Autodesk Inventor part; units mm, degrees
ref_plane "YZ Plane" through (0, 0, 0) normal (1, 0, 0) x (0, 1, 0)
ref_plane "XZ Plane" through (0, 0, 0) normal (0, 1, 0) x (-1, 0, 0)
ref_plane "XY Plane" through (0, 0, 0) normal (0, 0, 1) x (1, 0, 0)
sketch "Esboço1" plane through (0, 0, 0) normal (0, 0, 1) x (1, 0, 0)
  line L0 (0, 0) -> (75, 0)
  line L1 (75, 0) -> (75, 3)
  line L2 (75, 3) -> (0, 3)
  line L3 (0, 3) -> (0, 0)
  dimension "d0" = 75
  dimension "d1" = 3
revolve "Revolução1" add sketch "Esboço1" angle 360 about axis through (0, 0, 0) along (1, 0, 0)
sketch "Esboço2" plane through (0, 0, 0) normal (0, 1, 0) x (-1, 0, 0)
  point P0 (0, 0)
chamfer "Chanfro1" distance 0.5 angle 45 2 edges at (0, -3, 0) (75, -3, 0)
sketch "Esboço3" plane through (0, 0, 0) normal (0, 1, 0) x (-1, 0, 0)
  line L0 (0, 2.5) -> (0, -2.5)
  line L1 (-75, 2.5) -> (-74.5, 3)
  line L2 (-74.5, 3) -> (-0.5, 3)
  line L3 (-0.5, 3) -> (0, 2.5)
  line L4 (0, 2.5) -> (0, -2.5)
  line L5 (0, -2.5) -> (-0.5, -3)
  line L6 (-0.5, -3) -> (-74.5, -3)
  line L7 (-74.5, -3) -> (-75, -2.5)
  line L8 (-75, -2.5) -> (-75, 2.5)
  arc A0 (-9.5, -2) -> (-14.5, -2) centre (-12, -2) ccw
  line L9 (-65.5, 2) -> (-65.5, 3)
  line L10 (-60.5, 3) -> (-60.5, 2)
  arc A1 (-60.7087, 3) -> (-65.2913, 3) centre (-63, 2) ccw
  arc A2 (-65.5, 2) -> (-60.5, 2) centre (-63, 2) ccw
  line L11 (-65.5, 3) -> (-65.2913, 3)
  line L12 (-60.7087, 3) -> (-60.5, 3)
  line L13 (-75, 2.5) -> (-74.5, 3)
  line L14 (-74.5, 3) -> (-0.5, 3)
  line L15 (-0.5, 3) -> (0, 2.5)
  line L16 (0, 2.5) -> (0, -2.5)
  line L17 (0, -2.5) -> (-0.5, -3)
  line L18 (-0.5, -3) -> (-74.5, -3)
  line L19 (-74.5, -3) -> (-75, -2.5)
  line L20 (-75, -2.5) -> (-75, 2.5)
  line L21 (-0.5, -3) -> (-0.5, 3)
  line L22 (-74.5, 3) -> (-74.5, -3)
  line L23 (-75, 2.5) -> (-74.5, 3)
  line L24 (-74.5, 3) -> (-0.5, 3)
  line L25 (-0.5, 3) -> (0, 2.5)
  line L26 (0, 2.5) -> (0, -2.5)
  line L27 (0, -2.5) -> (-0.5, -3)
  line L28 (-0.5, -3) -> (-74.5, -3)
  line L29 (-74.5, -3) -> (-75, -2.5)
  line L30 (-75, -2.5) -> (-75, 2.5)
  line L31 (-14.5, -2) -> (-14.5, -5)
  line L32 (-14.5, -5) -> (-9.5, -5)
  line L33 (-9.5, -5) -> (-9.5, -2)
  point P0 (0, 0)
  point P1 (-14.5, -3)
  point P2 (-9.5, -3)
  point P3 (-14.5, -3)
  point P4 (-9.5, -3)
  dimension "d10" = 12
  dimension "d12" = 12
  dimension "d17" = 2.5
  dimension "d19" = 5
  dimension "d20" = 3
  dimension "d21" = 1
extrude "Extrusão1" cut sketch "Esboço3" against normal mid plane 1 contours L10 A2 L9 L2 | L6 L31 A0 L33 | L2 A1
properties part number "Mainpulo"
Geometry check sheet. Reference: the model listing, model coordinates, mm. A direction names the side the tool comes from. Coordinates: 2 decimals unless noted, no trailing zeros. Loops run counter-clockwise (first coordinate to the right, second up) from the corner with the lowest first, then second, coordinate; pieces in that order, holes last. Notation, with made-up numbers: (23.5, -29) - (77.5, -29) arc R18 ccw to (77.5, -13) - close; hole circle Ø4 at (48, 52). An arc over 180 degrees is marked (long way). One line per item, written item: value. Start each with the question number.
(1) Cross-section at A-A on x = 63. Enter the section's corners in (y, z).
(2) Cross-section at B-B on x = 50. Enter the section's corners in (y, z), plus the area to 3 significant figures.
(3) Material ranges on line 1 (Z direction, x = 52, y = -0.45); line 2 (Y direction, x = 26.5, z = 0.5); line 3 (X direction, y = -0.2, z = 1), recorded low to high. Write a range as [from, to].
(4) Depth check by flat-ended pin: P1, Ø1.5, axis at x = 37.5, z = 2, coming from the +Y side; P2, Ø3, axis at x = 37.5, z = -2, coming from the +Y side; P3, Ø1, axis at x = 12.5, z = -1.5, coming from the +Y side. Enter the tip coordinate at first touch or a pass-through.
(5) Cross-section at C-C on x = 12.5. Enter the section's corners in (y, z).
(6) Mould release check, pull along X, two halves, no side actions. Record for faces 1 (the flat face through (75, 0, 0)), 2 (the flat face through (0, 0, 0)), 3 (the cylindrical face through (11.9, 0, 0.5)): released by +X, released by -X, zero draft, split by the parting line, or undercut.
(7) Tool access check on faces 4 (the cylindrical face through (36.98, -0.65, 2.93)), 5 (the flat face through (12, -0.5, -2)), 6 (the flat face through (63, 0.5, 2)). Record the directions out of +Z, -Z, +X, -X, +Y, -Y that give a thin tool (end or side, any length) a straight path to the whole face; none if there is none.
Results below:
1. outline: (-0.5, -0.5) - (-0.5, 2.96) arc R3 ccw (long way) to (0.5, 2.96) - (0.5, -0.5) - close
2. outline: circle Ø6 at (0, 0)
2. area: 28.3 mm2
3. line 1: z = [-2.97, 2.97]
3. line 2: y = [-2.96, 2.96]
3. line 3: x = [0, 60.71], [65.29, 75]
4. P1: stops at y = 2.73
4. P2: stops at y = 2.96
4. P3: stops at y = 2.83
5. outline: (-0.5, -2.96) - (-0.5, 0.45) - (0.5, 0.45) - (0.5, -2.96) arc R3 ccw (long way) to start
6. face 1: released by +X
6. face 2: released by -X
6. face 3: undercut
7. face 4: +X, -X
7. face 5: -Z
7. face 6: +Z
